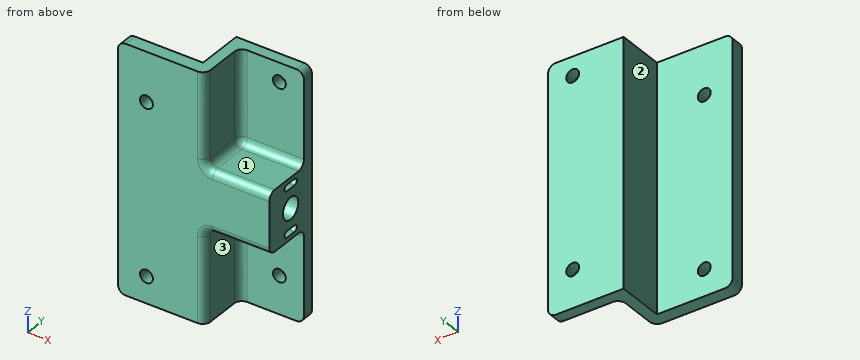
Autodesk Inventor part; units mm, degrees
ref_plane "YZ Plane" through (0, 0, 0) normal (1, 0, 0) x (0, 1, 0)
ref_plane "XZ Plane" through (0, 0, 0) normal (0, 1, 0) x (-1, 0, 0)
ref_plane "XY Plane" through (0, 0, 0) normal (0, 0, 1) x (1, 0, 0)
sketch "Sketch1" plane through (0, 0, 0) normal (0, 1, 0) x (-1, 0, 0)
  line L0 (0, 0) -> (40, 0)
  line L1 (40, 0) -> (40, -65)
  line L2 (40, -65) -> (0, -65)
  line L3 (0, -65) -> (0, 0)
  dimension "d0" = 40
  dimension "d1" = 65
extrude "Extrusion1" add sketch "Sketch1" along normal blind 16
sketch "Sketch2" plane through (-40, 0, 0) normal (0, 0, 1) x (1, 0, 0)
  line L0 (0, 16) -> (40, 16)
  line L1 (0, 16) -> (20, 16)
  line L2 (20, 16) -> (20, 3.5)
  line L3 (20, 3.5) -> (0, 3.5)
  line L4 (0, 3.5) -> (0, 16)
  line L5 (40, 0) -> (0, 0)
  dimension "d4" = 20
  dimension "d5" = 3.5
extrude "Extrusion2" cut sketch "Sketch2" against normal through all
sketch "Sketch3" plane through (0, 0, 0) normal (0, -1, 0) x (1, 0, 0)
  line L0 (-32.5, -58) -> (-32.5, -13) construction
  line L1 (-6.5, -55) -> (-6.5, -5) construction
  line L2 (-40, -65) -> (0, -65) construction
  line L3 (0, 0) -> (-40, 0) construction
  line L4 (0, -65) -> (0, 0) construction
  line L5 (-40, 0) -> (-40, -65) construction
  dimension "d8" = 45
  dimension "d9" = 50
  dimension "d10" = 7
  dimension "d11" = 5
  dimension "d12" = 6.5
  dimension "d13" = 7.5
hole "Hole1" at (-32.5, 0, -58) at (-32.5, 0, -13) at (-6.5, 0, -55) at (-6.5, 0, -5) direction (0, 1, 0) diameter 3.4 end through all
sketch "Sketch4" plane through (0, 0, 0) normal (1, 0, 0) x (0, 0, -1)
  line L0 (38.5, 6.5) -> (38.5, 9.5) construction
  line L1 (39.35, 6.5) -> (39.35, 9.5)
  line L2 (37.65, 9.5) -> (37.65, 6.5)
  arc A0 (37.65, 6.5) -> (39.35, 6.5) centre (38.5, 6.5) ccw
  arc A1 (39.35, 9.5) -> (37.65, 9.5) centre (38.5, 9.5) ccw
  line L3 (26.5, 6.5) -> (26.5, 9.5) construction
  line L4 (27.35, 6.5) -> (27.35, 9.5)
  line L5 (25.65, 9.5) -> (25.65, 6.5)
  arc A2 (25.65, 6.5) -> (27.35, 6.5) centre (26.5, 6.5) ccw
  arc A3 (27.35, 9.5) -> (25.65, 9.5) centre (26.5, 9.5) ccw
  line L6 (0, 0) -> (0, 16) construction
  line L7 (65, 0) -> (65, 16) construction
  line L8 (38.5, 8) -> (26.5, 8) construction
  line L9 (65, 0) -> (0, 0) construction
  line L10 (0, 16) -> (65, 16) construction
  line L11 (65, 0) -> (40.5, 0)
  line L12 (40.5, 0) -> (40.5, 13)
  line L13 (40.5, 13) -> (65, 13)
  line L14 (65, 13) -> (65, 0)
  line L15 (24.5, 0) -> (0, 0)
  line L16 (0, 0) -> (0, 13)
  line L17 (0, 13) -> (24.5, 13)
  line L18 (24.5, 13) -> (24.5, 0)
  point P0 (32.5, 8)
  dimension "d21" = 12
  dimension "d22" = 6
  dimension "d23" = 65
  dimension "d24" = 32.5
  dimension "d25" = 3
  dimension "d26" = 3
  dimension "d27" = 0.85
  dimension "d28" = 0.85
  dimension "d29" = 0
  dimension "d30" = 16
  dimension "d31" = 8
  dimension "d32" = 3
  dimension "d33" = 3
  dimension "d34" = 16
  dimension "d35" = 8
extrude "Extrusion3" cut sketch "Sketch4" against normal blind 2 contours A0 L2 A1 L1 | A2 L5 A3 L4
extrude "Extrusion4" cut sketch "Sketch4" against normal blind 17 contours L11 L12 L13 L14 | L15 L16 L17 L18
fillet "Fillet1" radius 2 14 edges at (-8.5, 0, -40.5) (-8.5, 0, -24.5) (-40, 1.75, -65) (-40, 1.75, 0) (0, 14.5, 0) (0, 14.5, -65) (-17, 0, -52.75) (-17, 0, -12.25) (-17, 6.5, -40.5) (-17, 6.5, -24.5) (-17, 13, -52.75) (-8.5, 13, -40.5) (-17, 13, -12.25) (-8.5, 13, -24.5)
hole "Hole2" at (0, 8, -32.5) direction (-1, 0, 0) diameter 5.75 depth 10 tip angle 118
equation "\"d26\" = d25"
equation "\"d28\" = d27"
properties part number "Dual Camera Mount"
For this review, take the finished solid that the model builds, in its own axes (mm). Face numbers are marked on the shaded views. A direction names the side the tool comes from. Give positions to 0.01 mm unless a question says otherwise; leave off trailing zeros. Write each loop counter-clockwise with the first axis right and the second up, starting at its lowest first coordinate (ties: lowest second). Pieces come first, ordered by that corner, then holes. Notation, with made-up numbers: M -27.75,-15 L 31.25,-15 A15 ccw 31.25,-11 Z; hole C 45,58.25 d10. An arc over 180 degrees is marked long. One line per item, written item: value.
1) Take a section at B-B, the plane y = 14. Write out the cut boundary in (x, z), then the cut area to 3 significant figures.
Results are:
outline: M -20,-65 L -2,-65 A2 ccw 0,-63 L 0,-2 A2 ccw -2,0 L -20,0 Z; hole C -6.5,-55 d3.4; hole C -6.5,-5 d3.4
area: 1,280 mm²
2) Take a section at D-D, the plane y = 4.5. Write out the cut boundary in (x, z).
Results are:
outline: M -20,-65 L -17,-65 L -17,-42.5 A2 cw -15,-40.5 L 0,-40.5 L 0,-24.5 L -15,-24.5 A2 cw -17,-22.5 L -17,0 L -20,0 Z
3) Take a section at C-C, the plane x = -32.5. Write out the cut boundary in (y, z).
Results are:
outline: M 0,-65 L 3.5,-65 L 3.5,-59.7 L 0,-59.7 Z; M 0,-56.3 L 3.5,-56.3 L 3.5,-14.7 L 0,-14.7 Z; M 0,-11.3 L 3.5,-11.3 L 3.5,0 L 0,0 Z
4) For line 1 (Z direction, x = -6.5, y = 14); line 2 (Z direction, x = -32.5, y = 2.65); line 3 (Y direction, x = -5.5, z = -32.5) (3 decimals), list the stretches that pass through material, from the lowest coordinate up. Write a range as from..to.
Results are:
line 1: z = -65..-56.7, -53.3..-6.7, -3.3..0
line 2: z = -65..-59.7, -56.3..-14.7, -11.3..0
line 3: y = 0..5.125, 10.875..16
5) Take a section at A-A, the plane z = -5. Write out the cut boundary in (x, y), then the cut area to 3 significant figures.
Results are:
outline: M -40,0 L -19,0 A2 ccw -17,2 L -17,11 A2 cw -15,13 L -8.2,13 L -8.2,16 L -20,16 L -20,3.5 L -40,3.5 Z; M -4.8,13 L 0,13 L 0,16 L -4.8,16 Z
area: 159 mm²
6) For P1, Ø5, axis at y = 8, z = -32.5, coming from the -X side; P2, Ø1, axis at x = -1.5, y = 8, coming from the +Z side; P3, Ø2, axis at x = -32.5, z = -13, coming from the +Y side; P4, Ø1, axis at x = -1.5, y = 8, coming from the -Z side, all flat-tipped, find the tip position at first contact; note any pin that passes through.
Results are:
P1: stops at x = -20
P2: stops at z = -24.5
P3: passes through
P4: stops at z = -40.5
7) For the marked faces 1, 2 and 3, list the 3-axis set-ups (+Z, -Z, +X, -X, +Y, -Y) from which the entire face can be reached by the end or side of a thin tool; tool diameter is ignored.
Results are:
face 1: +Z, +X, -Y
face 2: +Z, -Z, -X, +Y
face 3: -Z, +X, -Y
